```python
from build123d import *

# Parameters (mm, degrees)
F0_W      = 77.724
F0_H      = 35.687
F1_DEPTH  = 66.548
F2_T      = -1.524
F4_DEPTH  = 6.35
F5_DEPTH  = 25.4
F6_W      = 3.175
F6_H      = 6.35
F7_DEPTH  = 6.35
F8_W      = 3.175
F8_H      = 6.35
F9_DEPTH  = 6.35
F10_W     = 74.676
F10_H     = 63.5
F11_DEPTH = 1.524


with BuildPart() as f1:
    # F0 (on Top) → F1 (new body)
    with BuildSketch(Plane.XY):
        with Locations((38.862, 17.8435)):
            Rectangle(F0_W, F0_H)
    extrude(amount=F1_DEPTH)

    # F2 (hollow: no face is removed)
    offset(amount=F2_T, mode=Mode.SUBTRACT)

    # F3 (on face) → F4 (join)
    with BuildSketch(Plane.XY.offset(66.548)):
        Polygon((63.5, 14.224), (14.224, 14.224), (14.224, 35.687), (12.7, 35.687), (12.7, 12.7), (65.024, 12.7), (65.024, 35.687), (63.5, 35.687), align=None)
    extrude(amount=F4_DEPTH)

    # F5 (cut): a face of the model
    f5_faces = [f1.faces().sort_by_distance(p)[0] for p in [
        (38.862, 24.9555, 66.548),
    ]]
    extrude(f5_faces, amount=-F5_DEPTH, mode=Mode.SUBTRACT)

    # F6 (on face) → F7 (join)
    with BuildSketch(Plane.YZ.offset(77.724)):
        with Locations((34.0995, 15.875)):
            Rectangle(F6_W, F6_H)
        with Locations((34.0995, 50.673)):
            Rectangle(F6_W, F6_H)
    extrude(amount=F7_DEPTH)

    # F8 (on face) → F9 (join)
    with BuildSketch(Plane(origin=(0, 0, 0), x_dir=(0, -1, 0), z_dir=(-1, 0, 0))):
        with Locations((-34.0995, 15.875)):
            Rectangle(F8_W, F8_H)
        with Locations((-34.0995, 50.673)):
            Rectangle(F8_W, F8_H)
    extrude(amount=F9_DEPTH)

    # F10 (on face) → F11 (cut)
    with BuildSketch(Plane(origin=(0, 35.687, 0), x_dir=(-1, 0, 0), z_dir=(0, 1, 0))):
        with Locations((-38.862, 33.274)):
            Rectangle(F10_W, F10_H)
    extrude(amount=-F11_DEPTH, mode=Mode.SUBTRACT)


solid = f1.part
```
Input: part model. Units: mm. Frame: model coordinates. A direction names the side the tool comes from. Round coordinates to 2 decimals unless told otherwise and drop trailing zeros. Loops run counter-clockwise (first coordinate to the right, second up) from the corner with the lowest first, then second, coordinate; pieces in that order, holes last. Notation, with made-up numbers: M 37,71.5 L 75,71.5 A12 cw 75,79.5 Z; hole C 67,25.25 d2. An arc over 180 degrees is marked long. Answer in a Markdown table with one row per item. Add a question column.
1. Ray query, probe 1 along Z at (x, y) = (3.5, 2); probe 2 along X at (y, z) = (18, 29.5); probe 3 along Z at (x, y) = (1, 32). Return the intervals inside material, ascending.
2. Section A-A (y = 10.5). Output: boundary loops of the cut face in (x, z), and give its area (3 significant figures).
3. Contact query for flat-ended pins moving along their axis: pin 1 (5 mm diameter, centred on x = 66, z = 24, fed in from -Y); pin 2 (5 mm diameter, centred on x = 26.5, z = 55.5, fed in from +Y); pin 3 (1 mm diameter, centred on x = 81, y = 35, fed in from -Z); pin 4 (7 mm diameter, centred on x = 82, z = 51, fed in from -Y). Output: stop coordinate, or through.
4. Section D-D (y = 16.5). Output: boundary loops of the cut face in (x, z).
5. Mould query, pull axis X, two halves, no side actions, for faces 1 (the face through (39, 35.687, 1)), 2 (the face through (65.024, 24, 70)), 3 (the face through (14.224, 25, 69)). Classes: released by +X, released by -X, zero draft, split by the parting line, or undercut.
6. Section B-B (x = 73.5). Output: boundary loops of the cut face in (y, z), and give its area (3 significant figures).
7. Section C-C (z = 25). Output: boundary loops of the cut face in (x, y).
8. Set-up query: faces 4 (the face through (81, 34, 47.498)), 5 (the face through (39, 19, 1.524)), 6 (the face through (-3, 32.512, 16)), 7 (the face through (-3, 34, 12.7)). Return all of +Z, -Z, +X, -X, +Y, -Y with unobstructed straight access to the full face (end or side cutting, diameter ignored); none if empty.
Values follow:
| question | item | result |
|---|---|---|
| 1 | probe 1 | 0 to 1.52, 65.02 to 66.55 |
| 1 | probe 2 | 0 to 1.52, 76.2 to 77.72 |
| 1 | probe 3 | 0 to 66.55 |
| 2 | outline | M 0,0 L 77.72,0 L 77.72,66.55 L 0,66.55 Z; hole M 1.52,1.52 L 76.2,1.52 L 76.2,65.02 L 1.52,65.02 Z |
| 2 | area | 430 mm^2 |
| 3 | pin 1 | y = 0 |
| 3 | pin 2 | y = 1.52 |
| 3 | pin 3 | z = 12.7 |
| 3 | pin 4 | y = 32.51 |
| 4 | outline | M 0,0 L 77.72,0 L 77.72,66.55 L 65.02,66.55 L 65.02,72.9 L 63.5,72.9 L 63.5,65.02 L 76.2,65.02 L 76.2,1.52 L 1.52,1.52 L 1.52,65.02 L 14.22,65.02 L 14.22,72.9 L 12.7,72.9 L 12.7,66.55 L 0,66.55 Z |
| 5 | face 1 | zero draft |
| 5 | face 2 | released by +X |
| 5 | face 3 | undercut |
| 6 | outline | M 0,0 L 35.69,0 L 35.69,1.52 L 1.52,1.52 L 1.52,65.02 L 35.69,65.02 L 35.69,66.55 L 0,66.55 Z |
| 6 | area | 206 mm^2 |
| 7 | outline | M 0,0 L 77.72,0 L 77.72,35.69 L 76.2,35.69 L 76.2,1.52 L 1.52,1.52 L 1.52,35.69 L 0,35.69 Z |
| 8 | face 4 | +X, +Y, -Y |
| 8 | face 5 | +Y |
| 8 | face 6 | +Z, -Z, -X, -Y |
| 8 | face 7 | -Z, -X, +Y, -Y |
